Check sheet for the drawn part. Datum: minimum x, y, z corner. Units: mm. A direction names the side the tool comes from. Round coordinates to 2 decimals unless told otherwise and drop trailing zeros. Write each loop counter-clockwise with the first axis right and the second up, starting at its lowest first coordinate (ties: lowest second). Pieces come first, ordered by that corner, then holes. Notation, with made-up numbers: M -5.75,38.25 L 26.25,38.25 A16 cw 26.25,51.25 Z; hole C 65,-8 d2. An arc over 180 degrees is marked long. One line per item, written item: value. Start each with the question number.
Item 1: Draft check along X on the marked faces 1, 2, 3 and 4. Enter one of: +X half, -X half, draft (parallel to the pull), parting line (faces both ways), or undercut.
Item 2: Section check A-A, the plane x = 80.5. Record the cut outline in (y, z).
Item 3: Tool access check on the marked faces 5, 6, 7 and 8. Record the directions out of +Z, -Z, +X, -X, +Y, -Y that give a thin tool (end or side, any length) a straight path to the whole face; none if there is none.
Item 4: Section check D-D, the plane y = 41. Record the cut outline in (x, z).
Item 5: Gauge pin test, flat ends, axial feed: pin 1 (4 mm diameter, centred on y = 80, z = 6.5, fed in from -X); pin 2 (9 mm diameter, centred on y = 30.5, z = 21, fed in from +X); pin 3 (9 mm diameter, centred on y = 58, z = 12.5, fed in from -X); pin 4 (15 mm diameter, centred on x = 271, z = 8, fed in from -Y). Record the tip position at first contact, or that the pin passes through.
Item 6: Section check B-B, the plane y = 95.5. Record the cut outline in (x, z).
Item 7: Section check C-C, the plane z = 14. Record the cut outline in (x, y).
Item 8: Thickness scan on probe 1 along Y at (x, z) = (59, 23.5); probe 2 along Y at (x, z) = (244, 2); probe 3 along X at (y, z) = (73.5, 27). Record the ranges inside material, lowest first. Write a range as from..to.
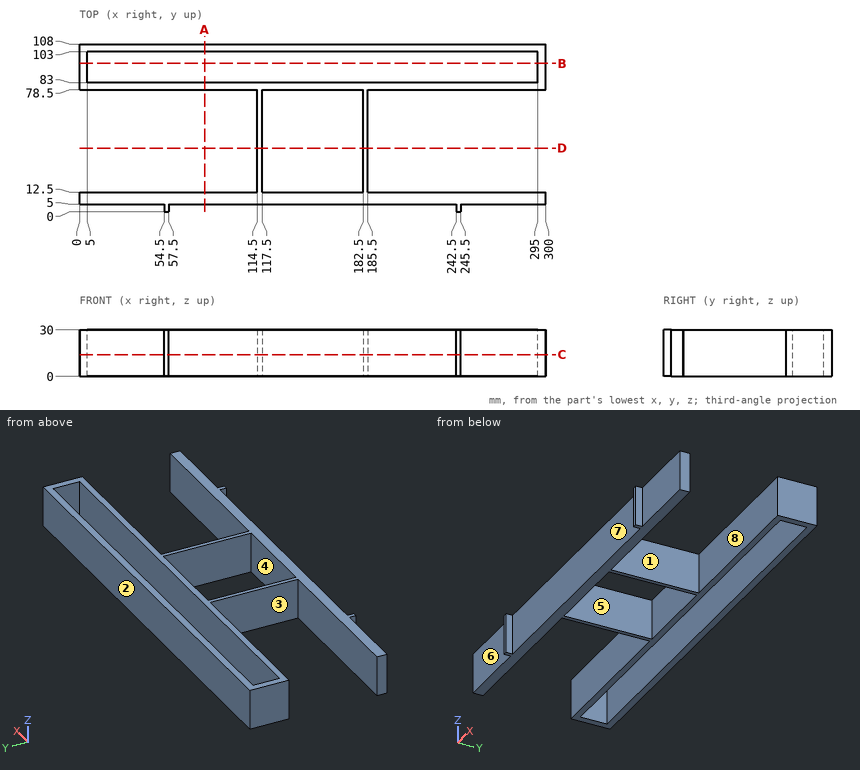
Response values:
1. face 1: +X half
1. face 2: draft
1. face 3: -X half
1. face 4: undercut
2. outline: M 5,0 L 12.5,0 L 12.5,30 L 5,30 Z; M 78.5,0 L 83,0 L 83,30 L 78.5,30 Z; M 103,0 L 108,0 L 108,30 L 103,30 Z
3. face 5: +Z, -Z
3. face 6: +Z, -Z, -X, -Y
3. face 7: +Z, -Z, -Y
3. face 8: +Z, -Z, +X
4. outline: M 114.5,0 L 117.5,0 L 117.5,30 L 114.5,30 Z; M 182.5,0 L 185.5,0 L 185.5,30 L 182.5,30 Z
5. pin 1: stops at x = 0
5. pin 2: stops at x = 185.5
5. pin 3: stops at x = 114.5
5. pin 4: stops at y = 5
6. outline: M 0,0 L 5,0 L 5,30 L 0,30 Z; M 295,0 L 300,0 L 300,30 L 295,30 Z
7. outline: M 0,5 L 54.5,5 L 54.5,0 L 57.5,0 L 57.5,5 L 242.5,5 L 242.5,0 L 245.5,0 L 245.5,5 L 300,5 L 300,12.5 L 185.5,12.5 L 185.5,78.5 L 300,78.5 L 300,108 L 0,108 L 0,78.5 L 114.5,78.5 L 114.5,12.5 L 0,12.5 Z; hole M 5,83 L 295,83 L 295,103 L 5,103 Z; hole M 117.5,12.5 L 182.5,12.5 L 182.5,78.5 L 117.5,78.5 Z
8. probe 1: y = 5..12.5, 78.5..83, 103..108
8. probe 2: y = 0..12.5, 78.5..83, 103..108
8. probe 3: x = 114.5..117.5, 182.5..185.5
